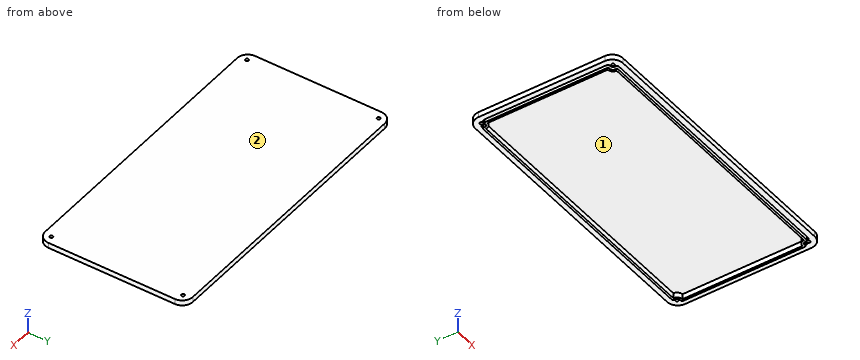
from build123d import *

# Parameters (mm, degrees)
SKETCH1_R           = 1.5
BOSS_EXTRUDE2_DEPTH = 3
BOSS_EXTRUDE3_DEPTH = 2
SKETCH3_R           = 1.5
CUT_EXTRUDE1_DEPTH  = 15.208
BOSS_EXTRUDE4_DEPTH = 5


with BuildPart() as part:
    # Sketch1 → Boss-Extrude2 (new body)
    with BuildSketch(Plane.XY):
        with BuildLine():
            Line((130, -70), (-130, -70))
            ThreePointArc((-130, -70), (-137.071067812, -67.071067812), (-140, -60))
            Line((-140, -60), (-140, 60))
            ThreePointArc((-140, 60), (-137.071067812, 67.071067812), (-130, 70))
            Line((-130, 70), (130, 70))
            ThreePointArc((130, 70), (137.071067812, 67.071067812), (140, 60))
            Line((140, 60), (140, -60))
            ThreePointArc((140, -60), (137.071067812, -67.071067812), (130, -70))
        make_face()
        with Locations((132.5, 62.5)):
            Circle(SKETCH1_R, mode=Mode.SUBTRACT)
        with Locations((-132.5, 62.5)):
            Circle(SKETCH1_R, mode=Mode.SUBTRACT)
        with Locations((-132.5, -62.5)):
            Circle(SKETCH1_R, mode=Mode.SUBTRACT)
        with Locations((132.5, -62.5)):
            Circle(SKETCH1_R, mode=Mode.SUBTRACT)
        with BuildLine():
            Line((130, 62), (130, 63))
            ThreePointArc((130, 63), (129.414213562, 64.414213562), (128, 65))
            Line((128, 65), (-128, 65))
            ThreePointArc((-128, 65), (-129.414213562, 64.414213562), (-130, 63))
            Line((-130, 63), (-130, 62))
            ThreePointArc((-130, 62), (-130.585786438, 60.585786438), (-132, 60))
            Line((-132, 60), (-133, 60))
            ThreePointArc((-133, 60), (-134.414213562, 59.414213562), (-135, 58))
            Line((-135, 58), (-135, -58))
            ThreePointArc((-135, -58), (-134.414213562, -59.414213562), (-133, -60))
            Line((-133, -60), (-132, -60))
            ThreePointArc((-132, -60), (-130.585786438, -60.585786438), (-130, -62))
            Line((-130, -62), (-130, -63))
            ThreePointArc((-130, -63), (-129.414213562, -64.414213562), (-128, -65))
            Line((-128, -65), (128, -65))
            ThreePointArc((128, -65), (129.414213562, -64.414213562), (130, -63))
            Line((130, -63), (130, -62))
            ThreePointArc((130, -62), (130.585786438, -60.585786438), (132, -60))
            Line((132, -60), (133, -60))
            ThreePointArc((133, -60), (134.414213562, -59.414213562), (135, -58))
            Line((135, -58), (135, 58))
            ThreePointArc((135, 58), (134.414213562, 59.414213562), (133, 60))
            Line((133, 60), (132, 60))
            ThreePointArc((132, 60), (130.585786438, 60.585786438), (130, 62))
        make_face(mode=Mode.SUBTRACT)
    extrude(amount=BOSS_EXTRUDE2_DEPTH)

    # Sketch2 → Boss-Extrude3 (add)
    with BuildSketch(Plane.XY.offset(3)):
        with BuildLine():
            Line((-130, -70), (130, -70))
            ThreePointArc((130, -70), (137.071067812, -67.071067812), (140, -60))
            Line((140, -60), (140, 60))
            ThreePointArc((140, 60), (137.071067812, 67.071067812), (130, 70))
            Line((130, 70), (-130, 70))
            ThreePointArc((-130, 70), (-137.071067812, 67.071067812), (-140, 60))
            Line((-140, 60), (-140, -60))
            ThreePointArc((-140, -60), (-137.071067812, -67.071067812), (-130, -70))
        make_face()
    extrude(amount=BOSS_EXTRUDE3_DEPTH)

    # Sketch3 → Cut-Extrude1 (cut)
    with BuildSketch(Plane(origin=(0, 0, 0), x_dir=(-1, 0, 0), z_dir=(0, 0, -1))):
        with Locations(Location((-132.5, -62.5, 0), (0, 0, 180))):
            Circle(SKETCH3_R)
        with Locations(Location((-132.5, 62.5, 0), (0, 0, 180))):
            Circle(SKETCH3_R)
        with Locations(Location((132.5, -62.5, 0), (0, 0, 180))):
            Circle(SKETCH3_R)
        with Locations(Location((132.5, 62.5, 0), (0, 0, 180))):
            Circle(SKETCH3_R)
    extrude(amount=-CUT_EXTRUDE1_DEPTH, mode=Mode.SUBTRACT)

    # Sketch4 → Boss-Extrude4 (add)
    with BuildSketch(Plane(origin=(0, 0, 3), x_dir=(-1, 0, 0), z_dir=(0, 0, -1))):
        with BuildLine():
            Line((129, 62), (129, 63))
            ThreePointArc((129, 63), (128.707106781, 63.707106781), (128, 64))
            Line((128, 64), (-128, 64))
            ThreePointArc((-128, 64), (-128.707106781, 63.707106781), (-129, 63))
            Line((-129, 63), (-129, 62))
            ThreePointArc((-129, 62), (-129.878679656, 59.878679656), (-132, 59))
            Line((-132, 59), (-133, 59))
            ThreePointArc((-133, 59), (-133.707106781, 58.707106781), (-134, 58))
            Line((-134, 58), (-134, -58))
            ThreePointArc((-134, -58), (-133.707106781, -58.707106781), (-133, -59))
            Line((-133, -59), (-132, -59))
            ThreePointArc((-132, -59), (-129.878679656, -59.878679656), (-129, -62))
            Line((-129, -62), (-129, -63))
            ThreePointArc((-129, -63), (-128.707106781, -63.707106781), (-128, -64))
            Line((-128, -64), (128, -64))
            ThreePointArc((128, -64), (128.707106781, -63.707106781), (129, -63))
            Line((129, -63), (129, -62))
            ThreePointArc((129, -62), (129.878679656, -59.878679656), (132, -59))
            Line((132, -59), (133, -59))
            ThreePointArc((133, -59), (133.707106781, -58.707106781), (134, -58))
            Line((134, -58), (134, 58))
            ThreePointArc((134, 58), (133.707106781, 58.707106781), (133, 59))
            Line((133, 59), (132, 59))
            ThreePointArc((132, 59), (129.878679656, 59.878679656), (129, 62))
        make_face()
        with BuildLine():
            Line((127, 62), (-127, 62))
            ThreePointArc((-127, 62), (-128.464466094, 58.464466094), (-132, 57))
            Line((-132, 57), (-132, -57))
            ThreePointArc((-132, -57), (-128.464466094, -58.464466094), (-127, -62))
            Line((-127, -62), (127, -62))
            ThreePointArc((127, -62), (128.464466094, -58.464466094), (132, -57))
            Line((132, -57), (132, 57))
            ThreePointArc((132, 57), (128.464466094, 58.464466094), (127, 62))
        make_face(mode=Mode.SUBTRACT)
    extrude(amount=BOSS_EXTRUDE4_DEPTH)


solid = part.part
Work out the finished part from the listing and answer in its coordinate system (mm). Face numbers are marked on the shaded views. Coordinates: 2 decimals unless noted, no trailing zeros. Order: outer loops, then holes, each group sorted by start corner. A loop starts at its lowest first (then second) coordinate and runs counter-clockwise, first axis right, second up. Notation, with made-up numbers: (66.5, 51) - (76.5, 51) arc R31 cw to (76.5, 88) - close; hole circle Ø2 at (61, 13). An arc over 180 degrees is marked (long way). Put each result on its own line as item: value. Start each with the question number.
1) Find section B-B (y = 49.5). Give the vertices of the cut face in (x, z), plus the area to 3 significant figures.
2) Find section A-A (z = 1.75). State how many separate pieces and enclosed holes the cut face has, plus the area to 3 significant figures.
3) Find the intervals of material crossed by line 1 (X direction, y = 32, z = 2.25); line 2 (Y direction, x = -80.5, z = 2); line 3 (X direction, y = -25.5, z = -0.75), in increasing order. Write a range as from..to.
4) For a pull along X with two mould halves and no side action, classify the marked faces 1 and 2 as released by +X, released by -X, zero draft, split by the parting line, or undercut.
5) Flat-ended cylindrical pins translate along their axes: pin 1 (0.5 mm diameter, centred on y = -62.5, z = 1, fed in from +X); pin 2 (1.5 mm diameter, centred on x = 39.5, y = 29, fed in from -Z); pin 3 (0.8 mm diameter, centred on x = 132.5, z = 1.5, fed in from +Y). Find the tip coordinate at first contact, or state that the pin passes through.
6) Find section C-C (x = -41.5). Give the vertices of the cut face in (y, z).
Results list:
1. outline: (-140, 0) - (-135, 0) - (-135, 3) - (-134, 3) - (-134, -2) - (-132, -2) - (-132, 3) - (132, 3) - (132, -2) - (134, -2) - (134, 3) - (135, 3) - (135, 0) - (140, 0) - (140, 5) - (-140, 5) - close
1. area: 610 mm^2
2. separate pieces: 2
2. enclosed holes: 6
2. area: 5,640 mm^2
3. line 1: x = -140..-135, -134..-132, 132..134, 135..140
3. line 2: y = -70..-65, -64..-62, 62..64, 65..70
3. line 3: x = -134..-132, 132..134
4. face 1: undercut
4. face 2: zero draft
5. pin 1: stops at x = 139.74
5. pin 2: stops at z = 3
5. pin 3: stops at y = 69.78
6. outline: (-70, 0) - (-65, 0) - (-65, 3) - (-64, 3) - (-64, -2) - (-62, -2) - (-62, 3) - (62, 3) - (62, -2) - (64, -2) - (64, 3) - (65, 3) - (65, 0) - (70, 0) - (70, 5) - (-70, 5) - close
